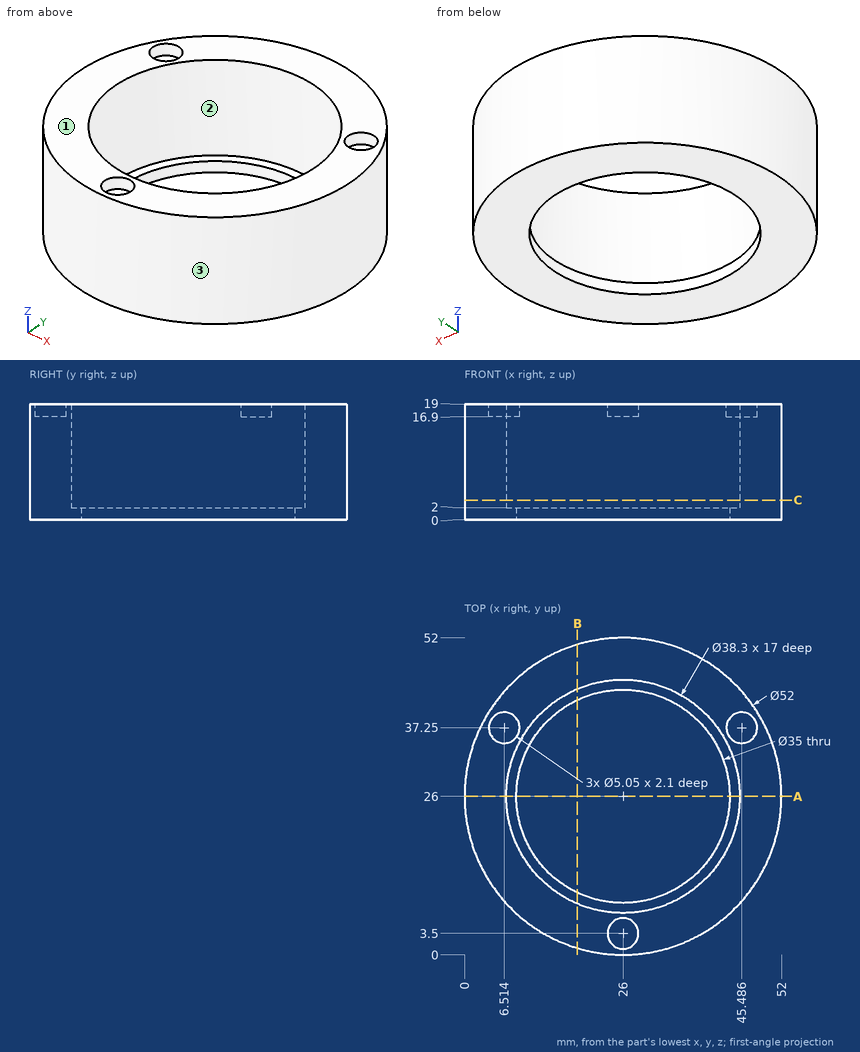
For this review, use the dimensioned drawing (mm, ordinates from the lowest corner) and the shaded views. Round coordinates to 2 decimals unless told otherwise and drop trailing zeros. Write each loop counter-clockwise with the first axis right and the second up, starting at its lowest first coordinate (ties: lowest second). Pieces come first, ordered by that corner, then holes. Notation, with made-up numbers: M -23.75,76.25 L -1.75,76.25 A26 cw -1.75,90.25 Z; hole C 74,43 d2. An arc over 180 degrees is marked long. Write item = value, one per line. Start each with the question number.
(1) For line 1 along Y through (x, z) = (25, 6.5); line 2 along Y through (x, z) = (18, 15.25); line 3 along X through (y, z) = (17.5, 1.75), list the stretches that pass through material, from the lowest coordinate up.
(2) We need section B-B (x = 18.5). Give the boundary of the cut face in (y, z) (1 decimal).
(3) The part is to be moulded in two halves that separate along X. For the marked faces 1, 2 and 3, say which applies: +X half, -X half, draft (parallel to the pull), parting line (faces both ways), or undercut.
(4) We need section C-C (z = 3.25). Give the boundary of the cut face in (x, y).
(5) Clearance check with flat-ended pins moving along their axes: pin 1 Ø1.5 at (y, z) = (17, 2) entering from -X; pin 2 Ø2.5 at (x, y) = (6.5, 36.5) entering from +Z; pin 3 Ø4 at (y, z) = (41.5, 3.5) entering from -X. State where each tip first meets the part, or that it passes through.
(6) We need section A-A (y = 26). Give the boundary of the cut face in (x, z), then the cut area to 3 significant figures.
Results found:
q1.line_1 = 0.02 to 6.88, 45.12 to 51.98
q1.line_2 = 1.26 to 8.6, 43.4 to 50.74
q1.line_3 = 1.43 to 10.7, 41.3 to 50.57
q2.outline = M 1.1,0 L 10.2,0 L 10.2,2 L 8.4,2 L 8.4,19 L 1.1,19 Z; M 41.8,0 L 50.9,0 L 50.9,19 L 43.6,19 L 43.6,2 L 41.8,2 Z
q3.face_1 = draft
q3.face_2 = undercut
q3.face_3 = parting line
q4.outline = C 26,26 d52; hole C 26,26 d38.3
q5.pin_1 = 1.34
q5.pin_2 = 16.9
q5.pin_3 = 3.78
q6.outline = M 0,0 L 8.5,0 L 8.5,2 L 6.85,2 L 6.85,19 L 0,19 Z; M 43.5,0 L 52,0 L 52,19 L 45.15,19 L 45.15,2 L 43.5,2 Z
q6.area = 267 mm²
